Autodesk Inventor part; units mm, degrees
ref_plane "Work Plane1" through (0, 12.7, 0) normal (0, 1, 0) x (-1, 0, 0)
ref_plane "YZ Plane" through (0, 0, 0) normal (1, 0, 0) x (0, 1, 0)
ref_plane "XY Plane" through (0, 0, 0) normal (0, 0, 1) x (1, 0, 0)
sketch "Sketch1" plane through (0, 0, 0) normal (0, 0, 1) x (1, 0, 0)
  circle A0 centre (0, 0) radius 12.7
  circle A1 centre (0, 0) radius 11.1125
  dimension "d0" = 25.4
  dimension "d1" = 22.225
extrude "Extrusion1" add sketch "Sketch1" along normal blind 393.7
ref_plane "Work Plane1" through (0, 12.7, 0) normal (0, 1, 0) x (-1, 0, 0)
sketch "Sketch2" plane through (0, 12.7, 0) normal (0, 1, 0) x (-1, 0, 0)
  line L0 (-12.7, 0) -> (-12.7, 393.7)
  line L1 (-12.7, 0) -> (12.7, 0)
  line L2 (12.7, 0) -> (12.7, 393.7)
  circle A0 centre (0, 6.35) radius 2.413
  circle A1 centre (0, 88.9) radius 2.413
  line L3 (0, 0) -> (0, 58.059) construction
  dimension "d4" = 4.826
  dimension "d6" = 6.35
  dimension "d7" = 88.9
extrude "Extrusion2" cut sketch "Sketch2" against normal blind 25.4
properties part number "Polycarbonate Clamp Tube 1 in OD (8585K14)" material "Polycarbonate, Clear"
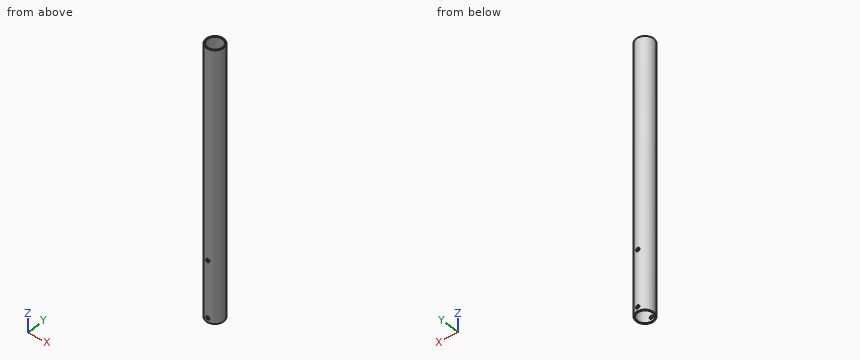
Check sheet for the modelled part. Datum: model origin and axes. Units: mm. Coordinates: 2 decimals unless noted, no trailing zeros. Write each loop counter-clockwise with the first axis right and the second up, starting at its lowest first coordinate (ties: lowest second). Pieces come first, ordered by that corner, then holes. Notation, with made-up numbers: M 52,8.5 L 92,8.5 A34 cw 92,43.5 Z; hole C -31.5,64 d2. An arc over 180 degrees is marked long. Use one line per item in the form item = value.
Item 1: Gauge pin test, flat ends, axial feed: pin 1 Ø6 at (x, z) = (5, 89) entering from +Y; pin 2 Ø3 at (y, z) = (2, 294) entering from -X; pin 3 Ø3 at (y, z) = (-5.5, 124) entering from -X; pin 4 Ø10 at (x, y) = (3, 0.5) entering from -Z. Record the tip position at first contact, or that the pin passes through.
Answer below:
pin_1 = 12.51
pin_2 = -12.69
pin_3 = -12.05
pin_4 = through
Item 2: Sectioned sample at B-B, the plane z = 141. Record the cut outline in (x, y) (1 decimal), and give its area (3 significant figures).
Answer below:
outline = C 0,0 d25.4; hole C 0,0 d22.2
area = 119 mm^2
Item 3: Material ranges on L1, parallel to Z at x = 0, y = -12; L2, parallel to X at y = -1, z = 262.5; L3, parallel to Y at x = 0, z = 205.5, recorded low to high. Write a range as from..to.
Answer below:
L1 = 0..3.94, 8.76..86.49, 91.31..393.7
L2 = -12.66..-11.07, 11.07..12.66
L3 = -12.7..-11.11, 11.11..12.7
Item 4: Sectioned sample at A-A, the plane y = 0. Record the cut outline in (x, z), and give its area (3 significant figures).
Answer below:
outline = M -12.7,0 L -11.11,0 L -11.11,393.7 L -12.7,393.7 Z; M 11.11,0 L 12.7,0 L 12.7,393.7 L 11.11,393.7 Z
area = 1,250 mm^2
